Source: CAD feature listing. Evaluate the final solid. Frame: model axes, mm. A direction names the side the tool comes from. Round coordinates to 2 decimals unless told otherwise and drop trailing zeros. Write each loop counter-clockwise with the first axis right and the second up, starting at its lowest first coordinate (ties: lowest second). Pieces come first, ordered by that corner, then holes.
from build123d import *

# Parameters (mm, degrees)
ESBO_O1_W                = 42.3
ESBO_O1_H                = 42.3
RESSALTO_EXTRUS_O1_DEPTH = 40
FILETE1_R                = 2.5
ESBO_O2_R                = 1.5
CORTE_EXTRUS_O2_DEPTH    = 4.5
ESBO_O3_R                = 11
RESSALTO_EXTRUS_O2_DEPTH = 2
ESBO_O4_R                = 2.5
RESSALTO_EXTRUS_O3_DEPTH = 24
ESBO_O5_W                = 8
ESBO_O5_H                = 1
CORTE_EXTRUS_O3_DEPTH    = 15


with BuildPart() as part:
    # Esboço1 → Ressalto-extrusão1 (new body)
    with BuildSketch(Plane.XY):
        Rectangle(ESBO_O1_W, ESBO_O1_H)
    extrude(amount=RESSALTO_EXTRUS_O1_DEPTH)

    # Filete1
    filete1_edges = [part.edges().sort_by_distance(p)[0] for p in [
        (-21.15, 21.15, 20),
        (21.15, 21.15, 20),
        (21.15, -21.15, 20),
        (-21.15, -21.15, 20),
    ]]
    fillet(filete1_edges, radius=FILETE1_R)

    # Esboço2 → Corte-extrusão2 (cut)
    with BuildSketch(Plane.XY.offset(40)):
        with Locations((-15.5, 15.5)):
            Circle(ESBO_O2_R)
        with Locations((15.5, 15.5)):
            Circle(ESBO_O2_R)
        with Locations((15.5, -15.5)):
            Circle(ESBO_O2_R)
        with Locations((-15.5, -15.5)):
            Circle(ESBO_O2_R)
    extrude(amount=-CORTE_EXTRUS_O2_DEPTH, mode=Mode.SUBTRACT)

    # Esboço3 → Ressalto-extrusão2 (add)
    with BuildSketch(Plane.XY.offset(40)):
        Circle(ESBO_O3_R)
    extrude(amount=RESSALTO_EXTRUS_O2_DEPTH)

    # Esboço4 → Ressalto-extrusão3 (add)
    with BuildSketch(Plane.XY.offset(42)):
        Circle(ESBO_O4_R)
    extrude(amount=RESSALTO_EXTRUS_O3_DEPTH)

    # Esboço5 → Corte-extrusão3 (cut)
    with BuildSketch(Plane.XY.offset(66)):
        with Locations((0, 2.5)):
            Rectangle(ESBO_O5_W, ESBO_O5_H)
    extrude(amount=-CORTE_EXTRUS_O3_DEPTH, mode=Mode.SUBTRACT)


solid = part.part
1) Section query D-D on x = 0. Return the cut outline in (y, z), then the cut area to 3 significant figures.
Taken from the geometry:
outline: (-21.15, 0) - (21.15, 0) - (21.15, 40) - (11, 40) - (11, 42) - (2.5, 42) - (2.5, 51) - (2, 51) - (2, 66) - (-2.5, 66) - (-2.5, 42) - (-11, 42) - (-11, 40) - (-21.15, 40) - close
area: 1,850 mm2
2) Pull-direction query (X, two-part tool) for faces 1 (the face through (-2.38, -10.74, 40.99)), 2 (the face through (-3, 0, 42)), 3 (the face through (-17, 15.57, 37.78)); classes: released by +X, released by -X, zero draft, split by the parting line, or undercut.
Taken from the geometry:
face 1: split by the parting line
face 2: zero draft
face 3: undercut
3) Section query C-C on z = 41. Return the cut outline in (x, y).
Taken from the geometry:
outline: circle Ø22 at (0, 0)
4) Material intervals for line 1 (Y direction, x = -15.5, z = 37.85); line 2 (X direction, y = -15, z = 38); line 3 (Z direction, x = -17, y = 17), sorted ascending.
Taken from the geometry:
line 1: y = -21.15 to -17, -14 to 14, 17 to 21.15
line 2: x = -21.15 to -16.91, -14.09 to 14.09, 16.91 to 21.15
line 3: z = 0 to 40
5) Contact query for flat-ended pins moving along their axis: P1, Ø0.9, axis at x = 16, y = -15.5, coming from the +Z side; P2, Ø3.5, axis at x = -15.5, y = 15.5, coming from the +Z side; P3, Ø5, axis at x = 2.5, z = 47, coming from the -Y side. Output: stop coordinate, or through.
Taken from the geometry:
P1: stops at z = 35.5
P2: stops at z = 40
P3: stops at y = -2.5
6) Section query A-A on x = -15.5. Return the cut outline in (y, z).
Taken from the geometry:
outline: (-21.15, 0) - (21.15, 0) - (21.15, 40) - (17, 40) - (17, 35.5) - (14, 35.5) - (14, 40) - (-14, 40) - (-14, 35.5) - (-17, 35.5) - (-17, 40) - (-21.15, 40) - close
7) Reachability of faces 4 (the face through (0, 2, 59)), 5 (the face through (-16, 16, 35.5)), 6 (the face through (0, 0, 0)) from +Z, -Z, +X, -X, +Y, -Y: full face, straight path, thin tool, end or side. Return the list, or none.
Taken from the geometry:
face 4: +Z, +X, -X, +Y
face 5: +Z
face 6: -Z, +X, -X, +Y, -Y
